```python
from build123d import *

# Parameters (mm, degrees)
EXTRUDE_1_DEPTH        = 7
EXTRUDE_1_DEPTH_BACK   = 7
SKETCH_1_W             = 15
SKETCH_1_H             = 34.3
EXTRUDE_1_2_DEPTH      = 7
EXTRUDE_1_2_DEPTH_BACK = 7
SKETCH_2_W             = 9.2
SKETCH_2_H             = 6.7
CUT_EXTRUDE_1_DEPTH    = 62
SKETCH_3_W             = 24
SKETCH_3_H             = 23.2
EXTRUDE_2_DEPTH        = 12
SKETCH_4_R             = 2.5
CUT_EXTRUDE_2_DEPTH    = 90
FILLET_1_R             = 2
CHAMFER_1_SIZE         = 5
CHAMFER_2_SIZE         = 5
FILLET_2_R             = 2
SKETCH_7_R             = 1.5
CUT_EXTRUDE_3_DEPTH    = 34
SKETCH_9_W             = 15
SKETCH_9_H             = 3
CUT_EXTRUDE_4_DEPTH    = 34


with BuildPart() as part:
    # Sketch 1 → Extrude 1 (new, two sides: drawn at the far end of the back side and taken through both)
    with BuildSketch(Plane.XY.offset(-EXTRUDE_1_DEPTH_BACK)):
        with Locations((30, 0)):
            Rectangle(SKETCH_1_W, SKETCH_1_H)
    extrude(amount=EXTRUDE_1_DEPTH + EXTRUDE_1_DEPTH_BACK)


with BuildPart() as body_2:
    # Sketch 1 → Extrude 1 2 (new, two sides: drawn at the far end of the back side and taken through both)
    with BuildSketch(Plane.XY.offset(-EXTRUDE_1_2_DEPTH_BACK)):
        with Locations((-30, 0)):
            Rectangle(SKETCH_1_W, SKETCH_1_H)
    extrude(amount=EXTRUDE_1_2_DEPTH + EXTRUDE_1_2_DEPTH_BACK)


with BuildPart() as cut_extrude_1_tool:
    # Sketch 2 → Cut-Extrude 1 (new body)
    with BuildSketch(Plane(origin=(0, 17.15, 0), x_dir=(1, 0, 0), z_dir=(0, 1, 0))):
        with Locations((30, 0)):
            Rectangle(SKETCH_2_W, SKETCH_2_H)
        with Locations((-30, 0)):
            Rectangle(SKETCH_2_W, SKETCH_2_H)
    extrude(amount=-CUT_EXTRUDE_1_DEPTH)


with BuildPart() as part_1:
    add(part.part)

    # Cut-Extrude 1: cut by cut_extrude_1_tool
    add(cut_extrude_1_tool.part, mode=Mode.SUBTRACT)



with BuildPart() as body_2_1:
    add(body_2.part)

    # Cut-Extrude 1: cut by cut_extrude_1_tool
    add(cut_extrude_1_tool.part, mode=Mode.SUBTRACT)


with BuildPart() as part_2:
    add(part_1.part)

    add(body_2_1.part)  # Extrude 2 merges body 2
    # Sketch 3 → Extrude 2 (add)
    with BuildSketch(Plane(origin=(0, 17.15, 0), x_dir=(1, 0, 0), z_dir=(0, 1, 0))):
        Polygon((22.5, 7), (17, 7), (17, 17.5), (-17, 17.5), (-17, 7), (-22.5, 7), (-22.5, -7), (-17, -7), (-17, -17.5), (17, -17.5), (17, -7), (22.5, -7), align=None)
        Rectangle(SKETCH_3_W, SKETCH_3_H, mode=Mode.SUBTRACT)
    extrude(amount=-EXTRUDE_2_DEPTH)

    # Sketch 4 → Cut-Extrude 2 (cut)
    with BuildSketch(Plane.XY.offset(17.5)):
        with Locations((0, 11.15)):
            Circle(SKETCH_4_R)
    extrude(amount=-CUT_EXTRUDE_2_DEPTH, mode=Mode.SUBTRACT)

    # Fillet 1
    fillet_1_edges = [part_2.edges().sort_by_distance(p)[0] for p in [
        (-37.5, 0, -7),
        (-37.5, 0, 7),
        (37.5, 0, 7),
        (37.5, 0, -7),
    ]]
    fillet(fillet_1_edges, radius=FILLET_1_R)

    # Chamfer 1
    chamfer_1_edges = [part_2.edges().sort_by_distance(p)[0] for p in [
        (22.5, 5.15, 0),
        (-22.5, 5.15, 0),
    ]]
    chamfer(chamfer_1_edges, length=CHAMFER_1_SIZE)

    # Chamfer 2
    # the kernel refuses this chamfer: 5 mm, written as the material it adds along each edge
    with BuildSketch(Plane(origin=(17, 17.15, -7), x_dir=(0.9996219169112968, 0, 0.027495876610586147), z_dir=(0, -1, 0))) as chamfer_2_piece_1_section:
        Polygon((CHAMFER_2_SIZE * 0.999621916911, -CHAMFER_2_SIZE * 0.0274958766106), (-CHAMFER_2_SIZE * 0.0274958766106, -CHAMFER_2_SIZE * 0.999621916911), (0, 0), align=None)
    chamfer_2_piece_1 = extrude(amount=12, mode=Mode.PRIVATE)
    chamfer_2_piece_1 = split(chamfer_2_piece_1, bisect_by=Plane(origin=(15.061953737, 7.588046263, -8.643148294), z_dir=(0.7071067811865476, 0.7071067811865475, 0)), keep=Keep.TOP, mode=Mode.PRIVATE)
    add(chamfer_2_piece_1)
    with BuildSketch(Plane(origin=(17, 17.15, -7), x_dir=(0.9996219169112968, 0, 0.027495876610586147), z_dir=(0, -1, 0))) as chamfer_2_piece_2_section:
        Polygon((CHAMFER_2_SIZE * 0.999621916911, -CHAMFER_2_SIZE * 0.0274958766106), (-CHAMFER_2_SIZE * 0.0274958766106, -CHAMFER_2_SIZE * 0.999621916911), (0, 0), align=None)
    chamfer_2_piece_2 = extrude(amount=12, mode=Mode.PRIVATE)
    chamfer_2_piece_2 = split(chamfer_2_piece_2, bisect_by=Plane(origin=(17.181894142, 5.468105858, -9.627776216), z_dir=(-0.7071067811865476, -0.7071067811865475, 0)), keep=Keep.TOP, mode=Mode.PRIVATE)
    add(chamfer_2_piece_2)
    with BuildSketch(Plane(origin=(17, 17.15, -7), x_dir=(0.9996219169112968, 0, 0.027495876610586147), z_dir=(0, -1, 0))) as chamfer_2_piece_3_section:
        Polygon((CHAMFER_2_SIZE * 0.999621916911, -CHAMFER_2_SIZE * 0.0274958766106), (-CHAMFER_2_SIZE * 0.0274958766106, -CHAMFER_2_SIZE * 0.999621916911), (0, 0), align=None)
    chamfer_2_piece_3 = extrude(amount=24.85841494, mode=Mode.PRIVATE)
    chamfer_2_piece_3 = split(chamfer_2_piece_3, bisect_by=Plane(origin=(19.269171179, 3.380828821, -8.010149173), z_dir=(0.7071067811865476, 0.7071067811865475, 0)), keep=Keep.TOP, mode=Mode.PRIVATE)
    chamfer_2_piece_3 = split(chamfer_2_piece_3, bisect_by=Plane(origin=(19.858894906, 5.15, -8.010149173), z_dir=(0, -1, 0)), keep=Keep.TOP, mode=Mode.PRIVATE)
    add(chamfer_2_piece_3)
    with BuildSketch(Plane(origin=(-17, 17.15, -7), x_dir=(0.027495876610586313, 0, -0.9996219169112968), z_dir=(0, -1, 0))) as chamfer_2_piece_4_section:
        Polygon((CHAMFER_2_SIZE * 0.999621916911, -CHAMFER_2_SIZE * 0.0274958766106), (-CHAMFER_2_SIZE * 0.0274958766106, -CHAMFER_2_SIZE * 0.999621916911), (0, 0), align=None)
    chamfer_2_piece_4 = extrude(amount=12, mode=Mode.PRIVATE)
    chamfer_2_piece_4 = split(chamfer_2_piece_4, bisect_by=Plane(origin=(-15.061953737, 7.588046263, -8.643148294), z_dir=(-0.7071067811865475, 0.7071067811865476, 0)), keep=Keep.TOP, mode=Mode.PRIVATE)
    add(chamfer_2_piece_4)
    with BuildSketch(Plane(origin=(-17, 17.15, -7), x_dir=(0.027495876610586313, 0, -0.9996219169112968), z_dir=(0, -1, 0))) as chamfer_2_piece_5_section:
        Polygon((CHAMFER_2_SIZE * 0.999621916911, -CHAMFER_2_SIZE * 0.0274958766106), (-CHAMFER_2_SIZE * 0.0274958766106, -CHAMFER_2_SIZE * 0.999621916911), (0, 0), align=None)
    chamfer_2_piece_5 = extrude(amount=24.85841494, mode=Mode.PRIVATE)
    chamfer_2_piece_5 = split(chamfer_2_piece_5, bisect_by=Plane(origin=(-19.858894906, 5.15, -8.010149173), z_dir=(0, -1, 0)), keep=Keep.TOP, mode=Mode.PRIVATE)
    chamfer_2_piece_5 = split(chamfer_2_piece_5, bisect_by=Plane(origin=(-19.269171179, 3.380828821, -8.010149173), z_dir=(-0.7071067811865475, 0.7071067811865476, 0)), keep=Keep.TOP, mode=Mode.PRIVATE)
    add(chamfer_2_piece_5)
    with BuildSketch(Plane(origin=(-17, 17.15, -7), x_dir=(0.027495876610586313, 0, -0.9996219169112968), z_dir=(0, -1, 0))) as chamfer_2_piece_6_section:
        Polygon((CHAMFER_2_SIZE * 0.999621916911, -CHAMFER_2_SIZE * 0.0274958766106), (-CHAMFER_2_SIZE * 0.0274958766106, -CHAMFER_2_SIZE * 0.999621916911), (0, 0), align=None)
    chamfer_2_piece_6 = extrude(amount=12, mode=Mode.PRIVATE)
    chamfer_2_piece_6 = split(chamfer_2_piece_6, bisect_by=Plane(origin=(-17.181894142, 5.468105858, -9.627776216), z_dir=(0.7071067811865475, -0.7071067811865476, 0)), keep=Keep.TOP, mode=Mode.PRIVATE)
    add(chamfer_2_piece_6)
    with BuildSketch(Plane(origin=(17, 17.15, 7), x_dir=(0.9996219169112968, 0, -0.027495876610586147), z_dir=(0, -1, 0))) as chamfer_2_piece_7_section:
        Polygon((CHAMFER_2_SIZE * 0.999621916911, CHAMFER_2_SIZE * 0.0274958766106), (-CHAMFER_2_SIZE * 0.0274958766106, CHAMFER_2_SIZE * 0.999621916911), (0, 0), align=None)
    chamfer_2_piece_7 = extrude(amount=12, mode=Mode.PRIVATE)
    chamfer_2_piece_7 = split(chamfer_2_piece_7, bisect_by=Plane(origin=(15.061953737, 7.588046263, 8.643148294), z_dir=(0.7071067811865476, 0.7071067811865475, 0)), keep=Keep.TOP, mode=Mode.PRIVATE)
    add(chamfer_2_piece_7)
    with BuildSketch(Plane(origin=(17, 17.15, 7), x_dir=(0.9996219169112968, 0, -0.027495876610586147), z_dir=(0, -1, 0))) as chamfer_2_piece_8_section:
        Polygon((CHAMFER_2_SIZE * 0.999621916911, CHAMFER_2_SIZE * 0.0274958766106), (-CHAMFER_2_SIZE * 0.0274958766106, CHAMFER_2_SIZE * 0.999621916911), (0, 0), align=None)
    chamfer_2_piece_8 = extrude(amount=12, mode=Mode.PRIVATE)
    chamfer_2_piece_8 = split(chamfer_2_piece_8, bisect_by=Plane(origin=(17.181894142, 5.468105858, 9.627776216), z_dir=(-0.7071067811865476, -0.7071067811865475, 0)), keep=Keep.TOP, mode=Mode.PRIVATE)
    add(chamfer_2_piece_8)
    with BuildSketch(Plane(origin=(17, 17.15, 7), x_dir=(0.9996219169112968, 0, -0.027495876610586147), z_dir=(0, -1, 0))) as chamfer_2_piece_9_section:
        Polygon((CHAMFER_2_SIZE * 0.999621916911, CHAMFER_2_SIZE * 0.0274958766106), (-CHAMFER_2_SIZE * 0.0274958766106, CHAMFER_2_SIZE * 0.999621916911), (0, 0), align=None)
    chamfer_2_piece_9 = extrude(amount=24.85841494, mode=Mode.PRIVATE)
    chamfer_2_piece_9 = split(chamfer_2_piece_9, bisect_by=Plane(origin=(19.269171179, 3.380828821, 8.010149173), z_dir=(0.7071067811865476, 0.7071067811865475, 0)), keep=Keep.TOP, mode=Mode.PRIVATE)
    chamfer_2_piece_9 = split(chamfer_2_piece_9, bisect_by=Plane(origin=(19.858894906, 5.15, 8.010149173), z_dir=(0, -1, 0)), keep=Keep.TOP, mode=Mode.PRIVATE)
    add(chamfer_2_piece_9)
    with BuildSketch(Plane(origin=(-17, 17.15, 7), x_dir=(0.027495876610586313, 0, 0.9996219169112968), z_dir=(0, -1, 0))) as chamfer_2_piece_10_section:
        Polygon((CHAMFER_2_SIZE * 0.999621916911, CHAMFER_2_SIZE * 0.0274958766106), (-CHAMFER_2_SIZE * 0.0274958766106, CHAMFER_2_SIZE * 0.999621916911), (0, 0), align=None)
    chamfer_2_piece_10 = extrude(amount=12, mode=Mode.PRIVATE)
    chamfer_2_piece_10 = split(chamfer_2_piece_10, bisect_by=Plane(origin=(-15.061953737, 7.588046263, 8.643148294), z_dir=(-0.7071067811865475, 0.7071067811865476, 0)), keep=Keep.TOP, mode=Mode.PRIVATE)
    add(chamfer_2_piece_10)
    with BuildSketch(Plane(origin=(-17, 17.15, 7), x_dir=(0.027495876610586313, 0, 0.9996219169112968), z_dir=(0, -1, 0))) as chamfer_2_piece_11_section:
        Polygon((CHAMFER_2_SIZE * 0.999621916911, CHAMFER_2_SIZE * 0.0274958766106), (-CHAMFER_2_SIZE * 0.0274958766106, CHAMFER_2_SIZE * 0.999621916911), (0, 0), align=None)
    chamfer_2_piece_11 = extrude(amount=24.85841494, mode=Mode.PRIVATE)
    chamfer_2_piece_11 = split(chamfer_2_piece_11, bisect_by=Plane(origin=(-19.858894906, 5.15, 8.010149173), z_dir=(0, -1, 0)), keep=Keep.TOP, mode=Mode.PRIVATE)
    chamfer_2_piece_11 = split(chamfer_2_piece_11, bisect_by=Plane(origin=(-19.269171179, 3.380828821, 8.010149173), z_dir=(-0.7071067811865475, 0.7071067811865476, 0)), keep=Keep.TOP, mode=Mode.PRIVATE)
    add(chamfer_2_piece_11)
    with BuildSketch(Plane(origin=(-17, 17.15, 7), x_dir=(0.027495876610586313, 0, 0.9996219169112968), z_dir=(0, -1, 0))) as chamfer_2_piece_12_section:
        Polygon((CHAMFER_2_SIZE * 0.999621916911, CHAMFER_2_SIZE * 0.0274958766106), (-CHAMFER_2_SIZE * 0.0274958766106, CHAMFER_2_SIZE * 0.999621916911), (0, 0), align=None)
    chamfer_2_piece_12 = extrude(amount=12, mode=Mode.PRIVATE)
    chamfer_2_piece_12 = split(chamfer_2_piece_12, bisect_by=Plane(origin=(-17.181894142, 5.468105858, 9.627776216), z_dir=(0.7071067811865475, -0.7071067811865476, 0)), keep=Keep.TOP, mode=Mode.PRIVATE)
    add(chamfer_2_piece_12)

    # Fillet 2
    fillet_2_edges = [part_2.edges().sort_by_distance(p)[0] for p in [
        (17, 11.15, 17.5),
        (-17, 11.15, 17.5),
        (-17, 11.15, -17.5),
        (17, 11.15, -17.5),
        (12, 11.15, 11.6),
        (-12, 11.15, 11.6),
        (-12, 11.15, -11.6),
        (12, 11.15, -11.6),
    ]]
    fillet(fillet_2_edges, radius=FILLET_2_R)

    # Sketch 7 → Cut-Extrude 3 (cut)
    with BuildSketch(Plane.XY.offset(7)):
        with Locations(Location((30, 11.8, 0), (0, 0, 180))):
            Circle(SKETCH_7_R)
        with Locations(Location((30, -8.2, 0), (0, 0, 180))):
            Circle(SKETCH_7_R)
        with Locations(Location((-30, -8.2, 0), (0, 0, 180))):
            Circle(SKETCH_7_R)
        with Locations(Location((-30, 11.8, 0), (0, 0, 180))):
            Circle(SKETCH_7_R)
    extrude(amount=-CUT_EXTRUDE_3_DEPTH, mode=Mode.SUBTRACT)

    # Sketch 9 → Cut-Extrude 4 (cut)
    with BuildSketch(Plane.XY.offset(7)):
        with Locations((-30, -15.65)):
            Rectangle(SKETCH_9_W, SKETCH_9_H)
        with Locations((30, -15.65)):
            Rectangle(SKETCH_9_W, SKETCH_9_H)
    extrude(amount=-CUT_EXTRUDE_4_DEPTH, mode=Mode.SUBTRACT)


solid = part_2.part
```
Input: part model. Units: mm. Frame: model coordinates. A direction names the side the tool comes from. Round coordinates to 2 decimals unless told otherwise and drop trailing zeros. Loops run counter-clockwise (first coordinate to the right, second up) from the corner with the lowest first, then second, coordinate; pieces in that order, holes last.
1) Section query A-A on y = -5. Return the cut outline in (x, z), plus the area to 3 significant figures.
Ans:
outline: (-37.5, -5) arc R2 ccw to (-35.5, -7) - (-22.5, -7) - (-22.5, 7) - (-35.5, 7) arc R2 ccw to (-37.5, 5) - close; (22.5, -7) - (35.5, -7) arc R2 ccw to (37.5, -5) - (37.5, 5) arc R2 ccw to (35.5, 7) - (22.5, 7) - close; hole (-34.6, -3.35) - (-25.4, -3.35) - (-25.4, 3.35) - (-34.6, 3.35) - close; hole (25.4, -3.35) - (34.6, -3.35) - (34.6, 3.35) - (25.4, 3.35) - close
area: 293 mm2
2) Pull-direction query (X, two-part tool) for faces 1 (the flat face through (20, 11, 9)), 2 (the flat face through (-34.6, 2, 0)), 3 (the flat face through (-37.5, 1, 0)); classes: released by +X, released by -X, zero draft, split by the parting line, or undercut.
Ans:
face 1: released by +X
face 2: undercut
face 3: released by -X
3) Pin query (flat end, axial travel): pin 1 (4 mm diameter, centred on y = 13, z = -14.5, fed in from +X); pin 2 (11 mm diameter, centred on x = 31.5, y = 1.5, fed in from -Z); pin 3 (4 mm diameter, centred on y = -6, z = 7.5, fed in from -X). Return the tip coordinate at first contact, or that it passes through.
Ans:
pin 1: stops at x = 17
pin 2: stops at z = -7
pin 3: stops at x = -37.44
4) Set-up query: faces 4 (the flat face through (-17, 11, -14)), 5 (the flat face through (29, 2, -7)), 6 (the cylindrical face through (11.4, 11.07, 11.03)). Return all of +Z, -Z, +X, -X, +Y, -Y with unobstructed straight access to the full face (end or side cutting, diameter ignored); none if empty.
Ans:
face 4: -Z, -X, +Y, -Y
face 5: -Z, +X, +Y, -Y
face 6: +Y, -Y
5) Section query D-D on y = 4. Return the cut outline in (x, z).
Ans:
outline: (-37.5, -5) arc R2 ccw to (-35.5, -7) - (-22, -7) - (-18.65, -10.35) - (-18.65, 10.35) - (-22, 7) - (-35.5, 7) arc R2 ccw to (-37.5, 5) - close; (18.65, -10.35) - (22, -7) - (35.5, -7) arc R2 ccw to (37.5, -5) - (37.5, 5) arc R2 ccw to (35.5, 7) - (22, 7) - (18.65, 10.35) - close; hole (-34.6, -3.35) - (-25.4, -3.35) - (-25.4, 3.35) - (-34.6, 3.35) - close; hole (25.4, -3.35) - (34.6, -3.35) - (34.6, 3.35) - (25.4, 3.35) - close
6) Section query C-C on x = -30. Return the cut outline in (y, z), plus the area to 3 significant figures.
Ans:
outline: (-14.15, -7) - (-9.7, -7) - (-9.7, -3.35) - (-14.15, -3.35) - close; (-14.15, 3.35) - (-9.7, 3.35) - (-9.7, 7) - (-14.15, 7) - close; (-6.7, -7) - (10.3, -7) - (10.3, -3.35) - (-6.7, -3.35) - close; (-6.7, 3.35) - (10.3, 3.35) - (10.3, 7) - (-6.7, 7) - close; (13.3, -7) - (17.15, -7) - (17.15, -3.35) - (13.3, -3.35) - close; (13.3, 3.35) - (17.15, 3.35) - (17.15, 7) - (13.3, 7) - close
area: 185 mm2
7) Material intervals for line 1 (X direction, y = -3, z = 1.5); line 2 (Y direction, x = 30, z = -4.9); line 3 (X direction, y = -8, z = 5), sorted ascending.
Ans:
line 1: x = -37.5 to -34.6, -25.4 to -22.5, 22.5 to 25.4, 34.6 to 37.5
line 2: y = -14.15 to -9.7, -6.7 to 10.3, 13.3 to 17.15
line 3: x = -37.5 to -31.49, -28.51 to -22.5, 22.5 to 28.51, 31.49 to 37.5
8) Section query B-B on x = 6.5. Return the cut outline in (y, z), plus the area to 3 significant figures.
Ans:
outline: (5.15, -17.5) - (17.15, -17.5) - (17.15, -11.6) - (5.15, -11.6) - close; (5.15, 11.6) - (17.15, 11.6) - (17.15, 17.5) - (5.15, 17.5) - close
area: 142 mm2
